Read the model definition and answer for the solid it produces. Units are mm, in the model's axes. Give positions to 0.01 mm unless a question says otherwise; leave off trailing zeros. Loops run counter-clockwise (first coordinate to the right, second up) from the corner with the lowest first, then second, coordinate; pieces in that order, holes last. Notation, with made-up numbers: (54, 46.25) - (87, 46.25) arc R18 cw to (87, 79.25) - close; hole circle Ø11 at (26.5, 22). An arc over 180 degrees is marked (long way). Use a Markdown table: item, result. Add a question column.
Item 1: A cutting plane is placed at B-B (z = 0.2). Determine the outline of the cut face in (x, y).
Item 2: A cutting plane is placed at A-A (z = 2.35). Determine the outline of the cut face in (x, y) (3 decimals).
Item 3: Consider probe 1 along Y at (x, z) = (0, 0.95); probe 2 along Y at (x, z) = (-0.75, 0.1); probe 3 along X at (y, z) = (1.25, 0.7). Determine where each line is inside the solid, lowest interval first. Write a range as [from, to].
Autodesk Fusion 360 part; units mm, degrees
sketch "Sketch1" plane through (0, 0, 0) normal (0, 0, 1) x (1, 0, 0) in component "Component"
  line L0 (1.875, 3.2476) -> (3.75, 0)
  line L1 (-1.875, 3.2476) -> (1.875, 3.2476)
  line L2 (-3.75, 0) -> (-1.875, 3.2476)
  line L3 (-1.875, -3.2476) -> (-3.75, 0)
  line L4 (1.875, -3.2476) -> (-1.875, -3.2476)
  line L5 (3.75, 0) -> (1.875, -3.2476)
extrude "Extrude1" add sketch "Sketch1" along normal blind 3.13 in component "Component"
sketch "Sketch2" plane through (0, 0, 0) normal (0, 0, 1) x (1, 0, 0) in component "Component"
  circle A0 centre (0, 0) radius 2.5
extrude "Extrude2" cut sketch "Sketch2" along normal through all in component "Component"
fillet "Fillet1" radius 0.3 1 edges at (-2.3308, 0.904, 3.13) in component "Component"
sketch "Sketch3" plane through (0, 0, 0) normal (0, 1, 0) x (1, 0, 0) in component "Component"
  line L0 (3.2476, 0) -> (3.75, 0)
  line L1 (3.75, 0) -> (3.75, -0.2901)
  line L2 (3.75, -0.2901) -> (3.2476, 0)
  line L3 (3.2476, -3.13) -> (3.75, -3.13)
  line L4 (3.75, -3.13) -> (3.75, -2.8399)
  line L5 (3.75, -2.8399) -> (3.2476, -3.13)
revolve "Revolve1" cut sketch "Sketch3" angle 360 about axis through (0, 0, 1.75) along (0, 0, 1) contours L3 L4 L5 in component "Component"
revolve "Revolve2" cut sketch "Sketch3" angle 360 about axis through (0, 0, 1.75) along (0, 0, 1) contours L0 L1 L2 in component "Component"
thread "Thread1" in component "Component"
component "Component" placed x (1, 0, 0) y (0, 1, 0) z (0, 0, 1) at (0, 0, 0)
Geometry says:
| question | item | result |
|---|---|---|
| 1 | outline | (-3.58, -0.29) - (-2.04, -2.96) arc R3.59 ccw to (-1.54, -3.25) - (1.54, -3.25) arc R3.59 ccw to (2.04, -2.96) - (3.58, -0.29) arc R3.59 ccw to (3.58, 0.29) - (2.04, 2.96) arc R3.59 ccw to (1.54, 3.25) - (-1.54, 3.25) arc R3.59 ccw to (-2.04, 2.96) - (-3.58, 0.29) arc R3.59 ccw to start; hole circle Ø5 at (0, 0) |
| 2 | outline | (-3.75, 0) - (-1.875, -3.248) - (1.875, -3.248) - (3.75, 0) - (1.875, 3.248) - (-1.875, 3.248) - close; hole circle Ø5 at (0, 0) |
| 3 | probe 1 | [-3.25, -2.5], [2.5, 3.25] |
| 3 | probe 2 | [-3.25, -2.38], [2.38, 3.25] |
| 3 | probe 3 | [-3.03, -2.17], [2.17, 3.03] |
